Geometry: final body of the model. Coordinates: model frame, mm. Face numbers are marked on the shaded views. A direction names the side the tool comes from. Give positions to 0.01 mm unless a question says otherwise; leave off trailing zeros. Write each loop counter-clockwise with the first axis right and the second up, starting at its lowest first coordinate (ties: lowest second). Pieces come first, ordered by that corner, then holes. Notation, with made-up numbers: M 73,11.25 L 105,11.25 A15 ccw 105,19.25 Z; hole C 65.5,89 d10. An arc over 180 degrees is marked long. Use a Markdown table: item, result. Add a question column.
(1) Reachability of the marked faces 1, 2 and 3 from +Z, -Z, +X, -X, +Y, -Y: full face, straight path, thin tool, end or side. Return the list, or none.
(2) Draft query along X for the marked faces 4, 5 and 6. Return one class per face: released by +X, released by -X, zero draft, split by the parting line, or undercut.
(3) Cut plane B-B (x = 2.75). Output: boundary loops of the cut face in (y, z).
(4) Cut plane D-D (y = 14). Output: boundary loops of the cut face in (x, z), plus the area to 3 significant figures.
(5) Material intervals for L1, parallel to Z at x = 10.25, y = 43, sorted ascending.
(6) Pin query (flat end, axial travel): pin 1 Ø4.5 at (x, y) = (4, 5.5) entering from +Z; pin 2 Ø1.5 at (x, z) = (5, 3) entering from +Y; pin 3 Ø0.6 at (x, y) = (19, 32.5) entering from +Z. Return the tip coordinate at first contact, or that it passes through.
(7) Cut plane C-C (y = 8). Output: boundary loops of the cut face in (x, z), plus the area to 3 significant figures.
(8) Cut plane A-A (z = 4.6). Output: boundary loops of the cut face in (x, y), plus the area to 3 significant figures.
```python
from build123d import *

# Parameters (mm, degrees)
F0_W      = 1.2
F0_H      = 49.8
F0_W_2    = 10
F1_DEPTH  = 0.12
F0_W_3    = 7
F0_H_2    = 0.1
F0_W_4    = 0.1
F1_FACE_W = 11.2
F1_FACE_H = 49.8
F2_DEPTH  = 0.1
F3_DEPTH  = 0.6
F4_W      = 10
F4_H      = 9
F4_W_2    = 0.1
F4_H_2    = 8.8
F5_DEPTH  = 2.5
F6_W      = 0.8
F6_H      = 2
F6_W_2    = 2
F6_H_2    = 1
F7_DEPTH  = 0.1
F8_W      = 0.8
F8_H      = 1.4
F8_H_2    = 2
F9_DEPTH  = 0.1
F11_DEPTH = 1
F12_W     = 10
F12_H     = 9
F12_W_2   = 3
F12_H_2   = 8.8
F13_DEPTH = 0.1
F14_W     = 10
F14_H     = 9
F14_W_2   = 9.8
F14_H_2   = 8.8
F15_DEPTH = 3
F16_W     = 1
F16_H     = 4
F17_DEPTH = 0.2
F18_W     = 0.1
F18_H     = 50
F19_DEPTH = 0.6
F21_DEPTH = 1


with BuildPart() as f1:
    # F0 (on Top) → F1 (new body)
    with BuildSketch(Plane.XY):
        with Locations((10.6, 25)):
            Rectangle(F0_W, F0_H)
        with Locations((5, 25)):
            Rectangle(F0_W_2, F0_H)
    extrude(amount=F1_DEPTH)



with BuildPart() as f1b:
    # F0 (on Top) → F1, piece 2 (new body)
    with BuildSketch(Plane.XY):
        with Locations((18.8, 25)):
            Rectangle(F0_W, F0_H)
    extrude(amount=F1_DEPTH)


with BuildPart() as f1_1:
    add(f1.part)

    add(f1b.part)  # F2 merges F1b
    # F0 (on Top) + F1_face (on face) → F2 (join)
    with BuildSketch(Plane.XY):
        with Locations((5, 25)):
            Rectangle(F0_W_2, F0_H)
        with Locations((10.6, 25)):
            Rectangle(F0_W, F0_H)
        with Locations((18.8, 25)):
            Rectangle(F0_W, F0_H)
        with Locations((14.7, 25)):
            Rectangle(F0_W_3, F0_H)
        with Locations((14.7, 0.05)):
            Rectangle(F0_W_3, F0_H_2)
        with Locations((10.6, 0.05)):
            Rectangle(F0_W, F0_H_2)
        with Locations((18.8, 0.05)):
            Rectangle(F0_W, F0_H_2)
        with Locations((19.45, 25)):
            Rectangle(F0_W_4, F0_H)
        with Locations((19.45, 0.05)):
            Rectangle(F0_W_4, F0_H_2)
        with Locations((5, 0.05)):
            Rectangle(F0_W_2, F0_H_2)
        with Locations((19.45, 49.95)):
            Rectangle(F0_W_4, F0_H_2)
        with Locations((18.8, 49.95)):
            Rectangle(F0_W, F0_H_2)
        with Locations((14.7, 49.95)):
            Rectangle(F0_W_3, F0_H_2)
        with Locations((10.6, 49.95)):
            Rectangle(F0_W, F0_H_2)
        with Locations((5, 49.95)):
            Rectangle(F0_W_2, F0_H_2)
    with BuildSketch(Plane(origin=(5.6, 25, 0.12), x_dir=(1, 0, 0), z_dir=(0, 0, 1))):
        Rectangle(F1_FACE_W, F1_FACE_H)
    extrude(amount=-F2_DEPTH)

    # F0 (on Top) → F3 (join)
    with BuildSketch(Plane.XY):
        with Locations((10.6, 49.95)):
            Rectangle(F0_W, F0_H_2)
        with Locations((5, 49.95)):
            Rectangle(F0_W_2, F0_H_2)
        with Locations((14.7, 49.95)):
            Rectangle(F0_W_3, F0_H_2)
        with Locations((18.8, 49.95)):
            Rectangle(F0_W, F0_H_2)
        with Locations((19.45, 25)):
            Rectangle(F0_W_4, F0_H)
        with Locations((19.45, 49.95)):
            Rectangle(F0_W_4, F0_H_2)
        with Locations((19.45, 0.05)):
            Rectangle(F0_W_4, F0_H_2)
        with Locations((18.8, 0.05)):
            Rectangle(F0_W, F0_H_2)
        with Locations((14.7, 0.05)):
            Rectangle(F0_W_3, F0_H_2)
        with Locations((5, 0.05)):
            Rectangle(F0_W_2, F0_H_2)
        with Locations((10.6, 0.05)):
            Rectangle(F0_W, F0_H_2)
    extrude(amount=F3_DEPTH)

    # F4 (on face) → F5 (join)
    with BuildSketch(Plane.XY.offset(0.12)):
        with Locations((5, 4.5)):
            Rectangle(F4_W, F4_H)
        Polygon((6.8, 0.1), (0.1, 0.1), (0.1, 8.9), (6.8, 8.9), (6.9, 8.9), (9.9, 8.9), (9.9, 0.1), (6.9, 0.1), align=None, mode=Mode.SUBTRACT)
        with Locations((6.85, 4.5)):
            Rectangle(F4_W_2, F4_H_2)
    extrude(amount=F5_DEPTH)

    # F6 (on face) → F7 (cut, through all)
    with BuildSketch(Plane.YZ.offset(10)):
        with Locations((1.4, 1.12)):
            Rectangle(F6_W, F6_H)
        with Locations((6, 1.62)):
            Rectangle(F6_W_2, F6_H_2)
    extrude(amount=-F7_DEPTH, mode=Mode.SUBTRACT)

    # F8 (on face) → F9 (cut, through all)
    with BuildSketch(Plane.YZ.offset(6.9)):
        with Locations((4.7, 0.82)):
            Rectangle(F8_W, F8_H)
        with Locations((6.5, 1.12)):
            Rectangle(F8_W, F8_H_2)
    extrude(amount=-F9_DEPTH, mode=Mode.SUBTRACT)

    # F10 (on face) → F11 (join)
    with BuildSketch(Plane.YZ.offset(0.1)):
        Polygon((0.1, 0.12), (3.8, 0.12), (3.8, 0.37), (3.5, 0.37), (3.5, 0.62), (3.2, 0.62), (3.2, 0.87), (2.9, 0.87), (2.9, 1.12), (2.6, 1.12), (2.6, 1.37), (2.3, 1.37), (2.3, 1.62), (2, 1.62), (2, 1.87), (1.7, 1.87), (1.7, 2.12), (1.4, 2.12), (1.4, 2.37), (1.1, 2.37), (1.1, 2.62), (0.1, 2.62), align=None)
    extrude(amount=F11_DEPTH)

    # F12 (on face) → F13 (join)
    with BuildSketch(Plane.XY.offset(2.62)):
        with Locations((5, 4.5)):
            Rectangle(F12_W, F12_H)
        Polygon((6.8, 8.9), (6.8, 0.1), (1.1, 0.1), (1.1, 1.1), (0.1, 1.1), (0.1, 8.9), align=None, mode=Mode.SUBTRACT)
        with Locations((8.4, 4.5)):
            Rectangle(F12_W_2, F12_H_2, mode=Mode.SUBTRACT)
        Polygon((1.1, 0.1), (6.8, 0.1), (6.8, 8.9), (0.1, 8.9), (0.1, 1.1), (1.1, 1.1), align=None)
        with Locations((8.4, 4.5)):
            Rectangle(F12_W_2, F12_H_2)
    extrude(amount=F13_DEPTH)

    # F14 (on face) → F15 (join)
    with BuildSketch(Plane.XY.offset(2.72)):
        with Locations((5, 4.5)):
            Rectangle(F14_W, F14_H)
        with Locations((5, 4.5)):
            Rectangle(F14_W_2, F14_H_2, mode=Mode.SUBTRACT)
    extrude(amount=F15_DEPTH)

    # F16 (on face) → F17 (cut)
    with BuildSketch(Plane.XY.offset(2.72)):
        with Locations((0.6, 2.1)):
            Rectangle(F16_W, F16_H)
    extrude(amount=-F17_DEPTH, mode=Mode.SUBTRACT)

    # F18 (on face) → F19 (join)
    with BuildSketch(Plane.XY):
        with Locations((0.05, 25)):
            Rectangle(F18_W, F18_H)
    extrude(amount=F19_DEPTH)

    # F20 (on face) → F21 (join)
    with BuildSketch(Plane.XY.offset(2.72)):
        Polygon((1.2, 4.2), (0.1, 4.2), (0.1, 4.1), (1.1, 4.1), (1.1, 1.1), (1.2, 1.1), align=None)
    extrude(amount=F21_DEPTH)


solid = f1_1.part
```
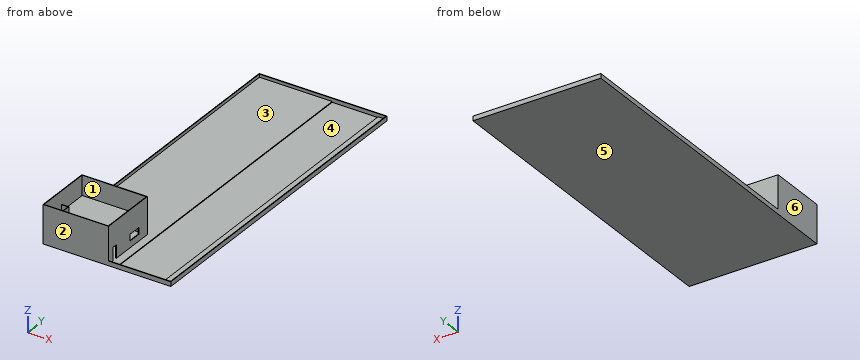
Answer list:
| question | item | result |
|---|---|---|
| 1 | face 1 | +Z |
| 1 | face 2 | +Z, -Z, +X, -X, -Y |
| 1 | face 3 | none |
| 2 | face 4 | undercut |
| 2 | face 5 | zero draft |
| 2 | face 6 | released by -X |
| 3 | outline | M 0,-0.1 L 50,-0.1 L 50,0.6 L 49.9,0.6 L 49.9,0.12 L 9,0.12 L 9,5.72 L 8.9,5.72 L 8.9,2.72 L 0.1,2.72 L 0.1,5.72 L 0,5.72 Z; hole M 0.1,0.12 L 8.9,0.12 L 8.9,2.62 L 0.1,2.62 Z |
| 4 | outline | M 0,-0.1 L 19.5,-0.1 L 19.5,0.6 L 19.4,0.6 L 19.4,0.12 L 18.2,0.12 L 18.2,0 L 11.2,0 L 11.2,0.12 L 0.1,0.12 L 0.1,0.6 L 0,0.6 Z |
| 4 | area | 3.55 mm² |
| 5 | L1 | -0.1 to 0.12 |
| 6 | pin 1 | z = 2.72 |
| 6 | pin 2 | y = 9 |
| 6 | pin 3 | z = 0.12 |
| 7 | outline | M 0,-0.1 L 19.5,-0.1 L 19.5,0.6 L 19.4,0.6 L 19.4,0.12 L 18.2,0.12 L 18.2,0 L 11.2,0 L 11.2,0.12 L 10,0.12 L 10,5.72 L 9.9,5.72 L 9.9,2.72 L 0.1,2.72 L 0.1,5.72 L 0,5.72 Z; hole M 0.1,0.12 L 6.8,0.12 L 6.8,2.62 L 0.1,2.62 Z; hole M 6.9,0.12 L 9.9,0.12 L 9.9,2.62 L 6.9,2.62 Z |
| 7 | area | 5.85 mm² |
| 8 | outline | M 0,0 L 10,0 L 10,9 L 0,9 Z; hole M 0.1,0.1 L 9.9,0.1 L 9.9,8.9 L 0.1,8.9 Z |
| 8 | area | 3.76 mm² |
